```python
from build123d import *

# Parameters (mm, degrees)
SKETCH_R  = 2.5
SKETCH_W  = 20.5
SKETCH_H  = 9
PAD_DEPTH = 2.5


with BuildPart() as part:
    # Sketch → Pad (new body)
    with BuildSketch(Plane.XY):
        with BuildLine():
            Line((-14.75, 10.5), (14.75, 10.5))
            Line((14.75, 10.5), (14.75, 3))
            ThreePointArc((14.75, -3), (27.016281, 0), (14.75, 3))
            Line((14.75, -10.5), (14.75, -3))
            Line((14.75, -10.5), (-14.75, -10.5))
            Line((-14.75, -3), (-14.75, -10.5))
            ThreePointArc((-14.75, 3), (-27.016281, 0), (-14.75, -3))
            Line((-14.75, 10.5), (-14.75, 3))
        make_face()
        with Locations((-20.516281, 0)):
            Circle(SKETCH_R, mode=Mode.SUBTRACT)
        with Locations((20.516281, 0)):
            Circle(SKETCH_R, mode=Mode.SUBTRACT)
        Rectangle(SKETCH_W, SKETCH_H, mode=Mode.SUBTRACT)
    extrude(amount=PAD_DEPTH)


solid = part.part
```
Read the model definition and answer for the solid it produces. Units are mm, in the model's axes. A direction names the side the tool comes from. Give positions to 0.01 mm unless a question says otherwise; leave off trailing zeros. Write each loop counter-clockwise with the first axis right and the second up, starting at its lowest first coordinate (ties: lowest second). Pieces come first, ordered by that corner, then holes. Notation, with made-up numbers: (-39, -37.75) -> (6, -37.75) arc R22 cw to (6, -25.75) -> close; hole circle Ø6 at (72.25, 16.25). An arc over 180 degrees is marked (long way). Answer as a JSON object with one key per item and string values.
1) Section B-B on z = 0.9 is taken. Write down the section's boundary in (x, y).
Findings below:
{"outline": "(-14.75, -10.5) -> (14.75, -10.5) -> (14.75, -3) arc R6.5 ccw (long way) to (14.75, 3) -> (14.75, 10.5) -> (-14.75, 10.5) -> (-14.75, 3) arc R6.5 ccw (long way) to (-14.75, -3) -> close; hole circle Ø5 at (-20.52, 0); hole (-10.25, -4.5) -> (10.25, -4.5) -> (10.25, 4.5) -> (-10.25, 4.5) -> close; hole circle Ø5 at (20.52, 0)"}
2) A tool of negligible diameter and unlimited length cuts with its end or side. For faces 1 (the flat face through (0, 5, 0)), 2 (the flat face through (-14.75, -7, 1)), 3 (the flat face through (0, -4.5, 1)), from which of +Z, -Z, +X, -X, +Y, -Y can it reach the whole face along a straight path? Write none if from no direction.
Findings below:
{"face 1": "-Z, +X, -X, +Y, -Y", "face 2": "+Z, -Z, -Y", "face 3": "+Z, -Z"}
3) Section C-C on y = -7.5 is taken. Write down the section's boundary in (x, z), then the cut area to 4 significant figures.
Findings below:
{"outline": "(-14.75, 0) -> (14.75, 0) -> (14.75, 2.5) -> (-14.75, 2.5) -> close", "area": "73.75 mm^2"}
4) Section D-D on x = -17 is taken. Write down the section's boundary in (y, z).
Findings below:
{"outline": "(-5.47, 0) -> (5.47, 0) -> (5.47, 2.5) -> (-5.47, 2.5) -> close"}
5) Straight lines are drawn through the part: probe 1 along Y at (x, z) = (-3.5, 0.3); probe 2 along X at (y, z) = (1.5, 2); probe 3 along X at (y, z) = (1, 1.9) (3 decimals). For each, find the intervals that lie inside material, in ascending order. Write a range as from..to.
Findings below:
{"probe 1": "y = -10.5..-4.5, 4.5..10.5", "probe 2": "x = -26.84..-22.52, -18.52..-10.25, 10.25..18.52, 22.52..26.84", "probe 3": "x = -26.939..-22.808, -18.225..-10.25, 10.25..18.225, 22.808..26.939"}
6) Section A-A on y = 0 is taken. Write down the section's boundary in (x, z).
Findings below:
{"outline": "(-27.02, 0) -> (-23.02, 0) -> (-23.02, 2.5) -> (-27.02, 2.5) -> close; (-18.02, 0) -> (-10.25, 0) -> (-10.25, 2.5) -> (-18.02, 2.5) -> close; (10.25, 0) -> (18.02, 0) -> (18.02, 2.5) -> (10.25, 2.5) -> close; (23.02, 0) -> (27.02, 0) -> (27.02, 2.5) -> (23.02, 2.5) -> close"}
7) For a pull along Y with two mould halves and no side action, classify faces 4 (the flat face through (10.25, 0, 1)), 5 (the flat face through (14.75, 7, 1)), 6 (the flat face through (0, 10.5, 1)) as pulls with the +Y half, pulls with the -Y half, needs draft (parallel to the pull), parting line crosses it, or undercut.
Findings below:
{"face 4": "undercut", "face 5": "needs draft", "face 6": "pulls with the +Y half"}
